Autodesk Inventor part; units mm, degrees
ref_plane "YZ Plane" through (0, 0, 0) normal (1, 0, 0) x (0, 1, 0)
ref_plane "XZ Plane" through (0, 0, 0) normal (0, 1, 0) x (-1, 0, 0)
ref_plane "XY Plane" through (0, 0, 0) normal (0, 0, 1) x (1, 0, 0)
sketch "Sketch1" plane through (0, 0, 0) normal (0, 0, 1) x (1, 0, 0)
  line L0 (-24, 7.25) -> (24, 7.25)
  line L1 (24, 7.25) -> (24, -7.25)
  line L2 (24, -7.25) -> (-24, -7.25)
  line L3 (-24, -7.25) -> (-24, 7.25)
  point P0 (0, 0)
  dimension "LENGTH" = 48
  dimension "WIDTH" = 14.5
  dimension "d0" = 7.25
  dimension "d3" = 24
extrude "Extrusion1" add sketch "Sketch1" along normal blind 5
sketch "Sketch3" plane through (0, 0, 5) normal (0, 0, 1) x (1, 0, 0)
  line L0 (-24, 7.25) -> (-24, -7.25)
  line L1 (24, -7.25) -> (24, 7.25)
  point P0 (0, 0)
  point P1 (-18, 0)
  point P2 (18, 0)
  dimension "d13" = 0
  dimension "d14" = 0
  dimension "d15" = 6
  dimension "d16" = 6
hole "Hole1" at (-18, 0, 5) at (18, 0, 5) direction (0, 0, -1) diameter 4.5 depth 5 counterbore diameter 8 counterbore depth 2
sketch "Sketch4" plane through (0, 0, 5) normal (0, 0, 1) x (1, 0, 0)
  line L0 (-13, 7.25) -> (13, 7.25)
  line L1 (13, 7.25) -> (13, -7.25)
  line L2 (13, -7.25) -> (-13, -7.25)
  line L3 (-13, -7.25) -> (-13, 7.25)
  point P0 (0, 0)
  dimension "d17" = 26
  dimension "d18" = 13
  dimension "d19" = 14.5
  dimension "d20" = 7.25
extrude "Extrusion2" add sketch "Sketch4" along normal blind 25
sketch "Sketch5" plane through (-24, 7.25, 0) normal (0, 1, 0) x (1, 0, 0)
  circle A0 centre (24, -19.05) radius 9.55
  line L0 (14.475, -19.05) -> (33.525, -19.05)
  line L1 (24, -28.6) -> (34.6, -28.6)
  line L2 (34.6, -28.6) -> (34.6, -9.5)
  line L3 (34.6, -9.5) -> (24, -9.5)
  line L4 (24, -9.5) -> (24, -28.6)
  circle A1 centre (24, -19.05) radius 10.05
  circle A2 centre (15.9891, -16.1343) radius 1.525
  circle A3 centre (15.9891, -21.9657) radius 1.525
  line L5 (24, -19.05) -> (15.9891, -16.1343)
  line L6 (15.9891, -21.9657) -> (24, -19.05)
  point P0 (24, 0)
  point P1 (24, -28.6)
  point P2 (24, -9.5)
  point P3 (15.5042, -14.6884)
  point P4 (14.5561, -15.6127)
  point P5 (14.5561, -22.4873)
  point P6 (15.5042, -23.4116)
  dimension "d23" = 0
  dimension "d24" = 19.05
  dimension "DIAMETER" = 19.1
  dimension "d26" = 0
  dimension "d30" = 10.6
  dimension "d31" = 0
  dimension "d32" = 9.55
  dimension "d33" = 9.55
  dimension "d48" = 20.1
  dimension "d49" = 3.05
  dimension "d50" = 3.05
  dimension "d51" = 20
  dimension "d52" = 20
  dimension "d53" = 8.525
  dimension "d54" = 8.525
extrude "Extrusion3" cut sketch "Sketch5" against normal blind 11.5 contours A0 L4 | A0 L3 A1 L1 | L4 L5 A2 A0 | A0 A3 L6 L4 | A2 A0 | A0 A2 | L3 L2 L1 A1 | L6 A3 A0 A2 L5 | A3 A0 | A0 A3 | A0 A3 A1 A2
fillet "Fillet1" radius 2 2 edges at (10.6, 1.5, 28.6) (10.6, 1.5, 9.5)
sketch "Sketch6" plane through (13, -7.25, 5) normal (1, 0, 0) x (0, 0, -1)
  line L0 (0, 14.5) -> (-25, 14.5)
  point P0 (5, 7.25)
  point P1 (-14.05, 8.75)
  dimension "d46" = 19.05
  dimension "d47" = 5.75
hole "Hole2" at (13, 1.5, 19.05) direction (-1, 0, 0) diameter 2.1565 depth 2.4
chamfer "Chamfer1" distance 1 angle 45 6 edges at (13, 0, 30) (-13, 0, 30) (-24, 7.25, 2.5) (-24, -7.25, 2.5) (24, 7.25, 2.5) (24, -7.25, 2.5)
sketch "Sketch7" plane through (0, 0, 0) normal (0, 0, -1) x (-1, 0, 0)
  line L0 (-5.5, 0) -> (-4.5, 0) construction
  line L1 (-5.5, -1.05) -> (-4.5, -1.05)
  line L2 (-4.5, 1.05) -> (-5.5, 1.05)
  arc A0 (-5.5, 1.05) -> (-5.5, -1.05) centre (-5.5, 0) ccw
  arc A1 (-4.5, -1.05) -> (-4.5, 1.05) centre (-4.5, 0) ccw
  point P0 (0, 0)
  point P1 (-5, 0)
  point P2 (5, 0)
  dimension "d58" = 1
  dimension "d59" = 1.05
  dimension "d60" = 10
  dimension "d61" = 0
  dimension "d62" = 0
  dimension "d63" = 5
hole "Hole3" at (-5, 0, 0) direction (0, 0, 1) diameter 2.1 depth 2.1
extrude "Extrusion4" cut sketch "Sketch7" against normal blind 2.1
sketch "Sketch8" plane through (-23, 7.25, 0) normal (0, 1, 0) x (1, 0, 0)
  circle A0 centre (23, 12.35) radius 12.7
  point P0 (23, 0)
  dimension "d73" = 0
  dimension "d74" = 12.35
  dimension "d75" = 25.4
extrude "Extrusion5" cut sketch "Sketch8" against normal up to surface (14.5 mm away)
equation "\"d19\" = WIDTH"
equation "\"d32\" = 0.5 * DIAMETER"
equation "\"d33\" = d32"
equation "\"d54\" = d53"
equation "\"TOLERANCE\" = 0.1"
equation "\"BEAM_HEIGHT\" = 19.05"
properties part number "RC04FC-F01-mount-01"
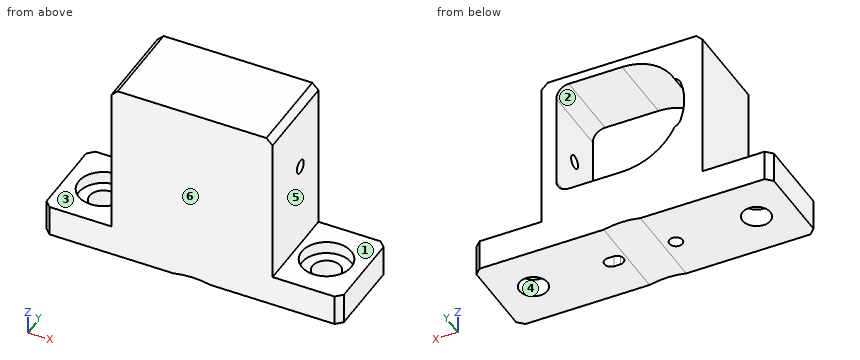
Check sheet for the modelled part. Datum: model origin and axes. Units: mm. Face numbers are marked on the shaded views. A direction names the side the tool comes from. Give positions to 0.01 mm unless a question says otherwise; leave off trailing zeros. Loops run counter-clockwise (first coordinate to the right, second up) from the corner with the lowest first, then second, coordinate; pieces in that order, holes last. Notation, with made-up numbers: M 58.5,-37 L 112.5,-37 A8 ccw 112.5,-26 Z; hole C 48.5,71 d2. An arc over 180 degrees is marked long. Use a Markdown table: item, result. Add a question column.
Q1. Sectioned sample at C-C, the plane x = 19.5. Record the cut outline in (y, z), then the cut area to 3 significant figures.
Q2. Sectioned sample at A-A, the plane y = 5. Record the cut outline in (x, z) (3 decimals), then the cut area to 3 significant figures.
Q3. Mould release check, pull along X, two halves, no side actions. Record for the marked faces 4, 5 and 6: pulls with the +X half, pulls with the -X half, needs draft (parallel to the pull), parting line crosses it, or undercut.
Q4. Scan lines: line 1 along X through (y, z) = (0, 0.9); line 2 along X through (y, z) = (0, 3.55); line 3 along Y through (x, z) = (-18, 4.5). Record each from-to range of solid material in increasing order. Write a range as [from, to].
Q5. Sectioned sample at D-D, the plane x = 0.5. Record the cut outline in (y, z), then the cut area to 3 significant figures.
Q6. Tool access check on the marked faces 1, 2 and 3. Record the directions out of +Z, -Z, +X, -X, +Y, -Y that give a thin tool (end or side, any length) a straight path to the whole face; none if there is none.
Q7. Sectioned sample at B-B, the plane z = 4.5. Record the cut outline in (x, y).
Q8. Go/stop test with flat-tipped pins: pin 1 (1.7 mm diameter, centred on x = -5, y = 0, fed in from -Z); pin 2 (8 mm diameter, centred on y = -3, z = 26, fed in from -X); pin 3 (5 mm diameter, centred on x = -18, y = 0, fed in from +Z). Record where each tip stops, or that it passes through.
Verdict:
| question | item | result |
|---|---|---|
| 1 | outline | M -7.25,0 L -1.68,0 L -1.68,3 L -3.71,3 L -3.71,5 L -7.25,5 Z; M 1.68,0 L 7.25,0 L 7.25,5 L 3.71,5 L 3.71,3 L 1.68,3 Z |
| 1 | area | 47.6 mm^2 |
| 2 | outline | M -24,0 L -2.961,0 A12.7 cw 2.961,0 L 24,0 L 24,5 L 13,5 L 13,29 L 12,30 L -12,30 L -13,29 L -13,5 L -24,5 Z; hole M -9.444,15.613 A1.525 ccw -8.496,14.688 A9.55 ccw 0,9.5 L 8.6,9.5 A2 ccw 10.6,11.5 L 10.6,26.6 A2 ccw 8.6,28.6 L 0,28.6 A9.55 ccw -8.496,23.412 A1.525 ccw -9.444,22.487 A10.05 ccw Z |
| 2 | area | 539 mm^2 |
| 3 | face 4 | undercut |
| 3 | face 5 | pulls with the +X half |
| 3 | face 6 | needs draft |
| 4 | line 1 | [-24, -20.25], [-15.75, -6.05], [-3.95, 3.45], [6.55, 15.75], [20.25, 24] |
| 4 | line 2 | [-24, -22], [-14, 14], [22, 24] |
| 4 | line 3 | [-7.25, -4], [4, 7.25] |
| 5 | outline | M -7.25,0.34 L 7.25,0.34 L 7.25,9.5 L -4.25,9.5 L -4.25,28.6 L 7.25,28.6 L 7.25,30 L -7.25,30 Z |
| 5 | area | 210 mm^2 |
| 6 | face 1 | +Z, +X, +Y, -Y |
| 6 | face 2 | +Y |
| 6 | face 3 | +Z, -X, +Y, -Y |
| 7 | outline | M -24,-6.25 L -23,-7.25 L 23,-7.25 L 24,-6.25 L 24,6.25 L 23,7.25 L -23,7.25 L -24,6.25 Z; hole C -18,0 d8; hole C 18,0 d8 |
| 8 | pin 1 | z = 2.1 |
| 8 | pin 2 | x = -13 |
| 8 | pin 3 | z = 3 |
